The figure shows three views and two pictorial views of one solid part (mm, origin at its lowest corner). Answer the questions. A direction names the side the tool comes from. Round coordinates to 2 decimals unless told otherwise and drop trailing zeros. Order: outer loops, then holes, each group sorted by start corner. A loop starts at its lowest first (then second) coordinate and runs counter-clockwise, first axis right, second up. Notation, with made-up numbers: (68.25, 38) -> (87.25, 38) arc R24 ccw to (87.25, 57) -> close; hole circle Ø6 at (66.25, -37). An arc over 180 degrees is marked (long way). Answer as a JSON object with one key per item and string values. Group by question number.
Item 1: Section C-C, the plane y = 6.25 is taken. Write down the section's boundary in (x, z).
Item 2: Section B-B, the plane x = 35.85 is taken. Write down the section's boundary in (y, z).
Item 3: Section A-A, the plane z = 18.4 is taken. Write down the section's boundary in (x, y).
Item 4: Consider probe 1 along X at (y, z) = (6, 19.5); probe 2 along X at (y, z) = (5.5, 4); probe 3 along Y at (x, z) = (26, 14). Determine where each line is inside the solid, lowest interval first. Write a range as from..to.
Item 5: Given P1, Ø4, axis at y = 7, z = 16.5, coming from the +X side; P2, Ø1, axis at x = 19.5, y = 5.5, coming from the +Z side; P3, Ø10, axis at x = 20.1, z = 18.4, coming from the -Y side, each flat-ended and moving along its own axis, determine where each tip first touches the part or whether it passes through.
Item 6: For the marked faces 1, 2 and 3, determine the directions among +Z, -Z, +X, -X, +Y, -Y from which every point of the face is accessible in a straight line to the end or side of a thin tool.
Item 7: Section D-D, the plane x = 20.1 is taken. Write down the section's boundary in (y, z), plus the area to 3 significant figures.
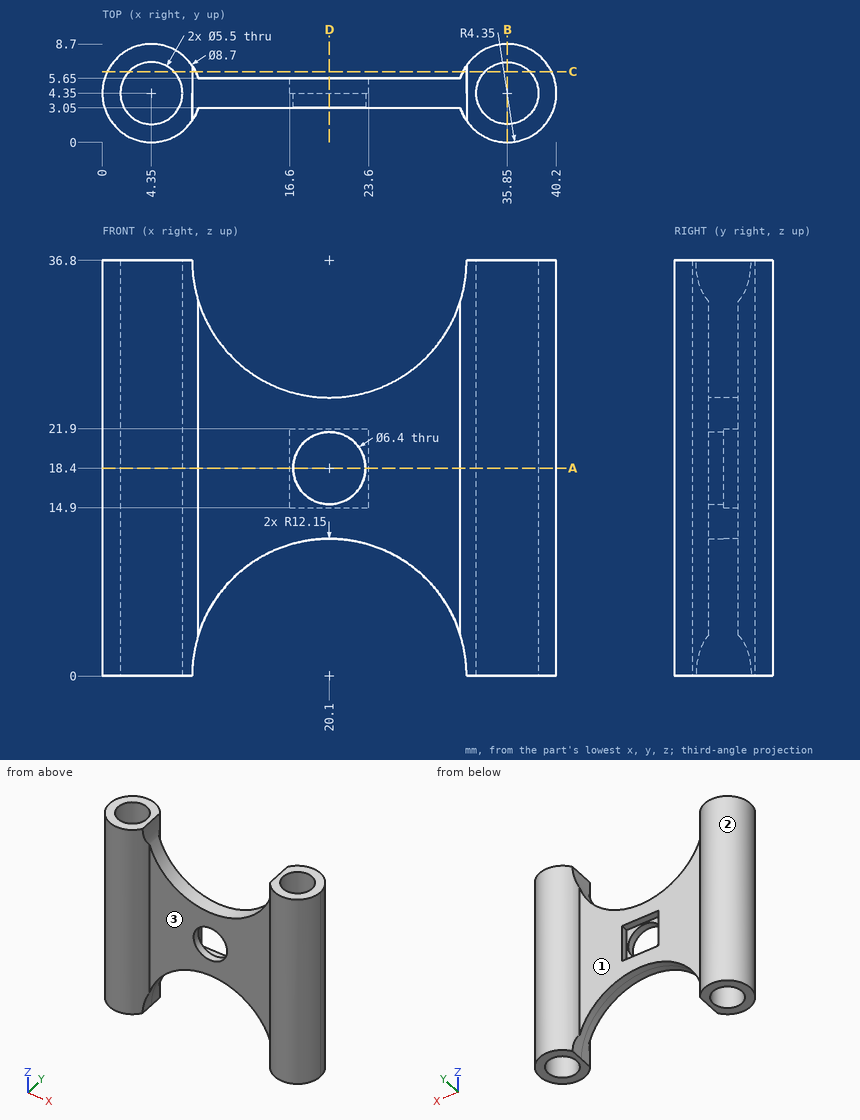
Values found:
{
 "1": {"outline": "(0.44, 0) -> (2.36, 0) -> (2.36, 36.8) -> (0.44, 36.8) -> close; (6.34, 0) -> (7.95, 0) arc R12.15 cw to (8.26, 2.74) -> (8.26, 34.06) arc R12.15 cw to (7.95, 36.8) -> (6.34, 36.8) -> close; (31.94, 2.74) arc R12.15 cw to (32.25, 0) -> (33.86, 0) -> (33.86, 36.8) -> (32.25, 36.8) arc R12.15 cw to (31.94, 34.06) -> close; (37.84, 0) -> (39.76, 0) -> (39.76, 36.8) -> (37.84, 36.8) -> close"},
 "2": {"outline": "(0, 0) -> (1.6, 0) -> (1.6, 36.8) -> (0, 36.8) -> close; (7.1, 0) -> (8.7, 0) -> (8.7, 36.8) -> (7.1, 36.8) -> close"},
 "3": {"outline": "(8.5, 3.05) -> (16.9, 3.05) -> (16.9, 4.35) -> (16.6, 4.35) -> (16.6, 5.65) -> (8.5, 5.65) arc R4.35 ccw (long way) to start; (23.3, 3.05) -> (31.7, 3.05) arc R4.35 ccw (long way) to (31.7, 5.65) -> (23.6, 5.65) -> (23.6, 4.35) -> (23.3, 4.35) -> close; hole circle Ø5.5 at (4.35, 4.35); hole circle Ø5.5 at (35.85, 4.35)"},
 "4": {"probe 1": "0.33..2.15, 6.55..8.37, 31.83..33.65, 38.05..39.87", "probe 2": "0.15..1.85, 6.85..8.63, 31.57..33.35, 38.35..40.05", "probe 3": "3.05..5.65"},
 "5": {"P1": "x = 40.15", "P2": "z = 24.7", "P3": "y = 3.05"},
 "6": {"face 1": "+Z, -Z, +Y", "face 2": "+Z, -Z", "face 3": "+Z, -Z, -Y"},
 "7": {"outline": "(3.05, 12.15) -> (5.65, 12.15) -> (5.65, 14.9) -> (4.35, 14.9) -> (4.35, 15.2) -> (3.05, 15.2) -> close; (3.05, 21.6) -> (4.35, 21.6) -> (4.35, 21.9) -> (5.65, 21.9) -> (5.65, 24.65) -> (3.05, 24.65) -> close", "area": "15.1 mm2"}
}
